```python
from build123d import *

# Parameters (mm, degrees)
SKETCH1_W               = 200
SKETCH1_H               = 100
BOSS_EXTRUDE1_DEPTH     = 2.6
FILLET1_R               = 10
SKETCH6_R               = 1.5
CUT_EXTRUDE6_DEPTH      = 2.6
MIRROR6_COPY_1_SKETCH_R = 1.5
MIRROR6_COPY_1_DEPTH    = 2.6
SKETCH15_R              = 10
CUT_EXTRUDE14_DEPTH     = 224.621913059
SKETCH20_R              = 1.27
CUT_EXTRUDE15_DEPTH     = 224.621913059
SKETCH23_R              = 1.524
CUT_EXTRUDE16_DEPTH     = 2.59999988
MIRROR8_COPY_1_SKETCH_R = 1.524
MIRROR8_COPY_1_DEPTH    = 2.59999988


with BuildPart() as part:
    # Sketch1 → Boss-Extrude1 (new body)
    with BuildSketch(Plane(origin=(0, 0, 0), x_dir=(1, 0, 0), z_dir=(0, 1, 0))):
        with Locations((100, -50)):
            Rectangle(SKETCH1_W, SKETCH1_H)
    extrude(amount=BOSS_EXTRUDE1_DEPTH)

    # Fillet1
    fillet1_edges = [part.edges().sort_by_distance(p)[0] for p in [
        (0, 1.3, 0),
        (200, 1.3, 0),
        (200, 1.3, 100),
        (0, 1.3, 100),
    ]]
    fillet(fillet1_edges, radius=FILLET1_R)

    # Sketch6 → Cut-Extrude6 (cut)
    with BuildSketch(Plane.XZ):
        with Locations(Location((190, 10, 0), (0, 0, 270))):
            Circle(SKETCH6_R)
    cut_extrude6 = extrude(amount=-CUT_EXTRUDE6_DEPTH, mode=Mode.SUBTRACT)

    # Mirror5: Cut-Extrude6 across plane
    add(cut_extrude6.mirror(Plane(origin=(100, 0, 0), x_dir=(0, 0, 1), z_dir=(1, 0, 0))), mode=Mode.SUBTRACT)

    # Mirror6: Cut-Extrude6 across plane
    add(cut_extrude6.mirror(Plane.XY.offset(50)), mode=Mode.SUBTRACT)

    # Mirror6 copy 1 sketch → Mirror6 copy 1 (cut)
    with BuildSketch(Plane(origin=(200, 0, 100), x_dir=(-1, 0, 0), z_dir=(0, -1, 0))):
        with Locations(Location((190, 10, 0), (0, 0, 270))):
            Circle(MIRROR6_COPY_1_SKETCH_R)
    extrude(amount=-MIRROR6_COPY_1_DEPTH, mode=Mode.SUBTRACT)

    # Sketch15 → Cut-Extrude14 (cut, through all)
    with BuildSketch(Plane.XZ):
        with Locations(Location((100, 50, 0), (0, 0, 270))):
            Circle(SKETCH15_R)
    extrude(amount=-CUT_EXTRUDE14_DEPTH, mode=Mode.SUBTRACT)

    # Sketch20 → Cut-Extrude15 (cut, through all)
    with BuildSketch(Plane(origin=(0, 2.6, 0), x_dir=(1, 0, 0), z_dir=(0, 1, 0))):
        with Locations(Location((158.41, -42.38, 0), (0, 0, 270))):
            Circle(SKETCH20_R)
        with Locations(Location((180, -42.38, 0), (0, 0, 270))):
            Circle(SKETCH20_R)
        with Locations(Location((158.41, -57.62, 0), (0, 0, 270))):
            Circle(SKETCH20_R)
        with Locations(Location((180, -57.62, 0), (0, 0, 270))):
            Circle(SKETCH20_R)
    extrude(amount=-CUT_EXTRUDE15_DEPTH, mode=Mode.SUBTRACT)

    # Sketch23 → Cut-Extrude16 (cut)
    with BuildSketch(Plane(origin=(0, 2.6, 0), x_dir=(1, 0, 0), z_dir=(0, 1, 0))):
        with Locations(Location((18.288, -9.906, 0), (0, 0, 270))):
            Circle(SKETCH23_R)
    cut_extrude16 = extrude(amount=-CUT_EXTRUDE16_DEPTH, mode=Mode.SUBTRACT)

    # Mirror7: Cut-Extrude16 across plane
    add(cut_extrude16.mirror(Plane(origin=(100, 0, 0), x_dir=(0, 0, 1), z_dir=(1, 0, 0))), mode=Mode.SUBTRACT)

    # Mirror8: Cut-Extrude16 across plane
    add(cut_extrude16.mirror(Plane.XY.offset(50)), mode=Mode.SUBTRACT)

    # Mirror8 copy 1 sketch → Mirror8 copy 1 (cut)
    with BuildSketch(Plane(origin=(200, 2.6, 100), x_dir=(-1, 0, 0), z_dir=(0, 1, 0))):
        with Locations(Location((18.288, -9.906, 0), (0, 0, 270))):
            Circle(MIRROR8_COPY_1_SKETCH_R)
    extrude(amount=-MIRROR8_COPY_1_DEPTH, mode=Mode.SUBTRACT)


solid = part.part
```
Check sheet for the modelled part. Datum: model origin and axes. Units: mm. Round coordinates to 2 decimals unless told otherwise and drop trailing zeros. Loops run counter-clockwise (first coordinate to the right, second up) from the corner with the lowest first, then second, coordinate; pieces in that order, holes last. Notation, with made-up numbers: (33.5, 44) - (50.5, 44) arc R38 ccw to (50.5, 83) - close; hole circle Ø9 at (-27.75, 55). An arc over 180 degrees is marked (long way). Write item = value, one per line. Start each with the question number.
Q1. Thickness scan on L1, parallel to X at y = 1.5, z = 10; L2, parallel to Z at x = 10, y = 1.5; L3, parallel to Z at x = 180, y = 1.75. Record the ranges inside material, lowest first.
Q2. Section check C-C (y = 1.6). Count the separate pieces of the cut face and the enclosed holes in it, plus the area to 3 significant figures.
Q3. Depth check by flat-ended pin: P1, Ø3.5, axis at x = 10, z = 90, coming from the -Y side; P2, Ø1.8, axis at x = 10, z = 10, coming from the -Y side. Enter the tip coordinate at first touch or a pass-through.
Q4. Section check B-B (z = 50). Record the boundary of the cut face in (x, y).
Q5. Release check for a two-part mould opening along Z. For faces 1 (the face through (2.85, 1.32, 96.99)), 2 (the face through (109.915, 1.282, 51.302)), 3 (the face through (99, 0, 38)) record: pulls with the +Z half, pulls with the -Z half, needs draft (parallel to the pull), parting line crosses it, or undercut.
Q6. Section check A-A (x = 100). Record the boundary of the cut face in (y, z), plus the area to 3 significant figures.
Derived:
q1.L1 = 0 to 8.5, 11.5 to 16.77, 19.81 to 180.19, 183.23 to 188.5, 191.5 to 200
q1.L2 = 0 to 8.5, 11.5 to 88.5, 91.5 to 100
q1.L3 = 0 to 41.11, 43.65 to 56.35, 58.89 to 100
q2.separate_pieces = 1
q2.enclosed_holes = 13
q2.area = 19,500 mm^2
q3.P1 = 0
q3.P2 = through
q4.outline = (0, 0) - (90, 0) - (90, 2.6) - (0, 2.6) - close; (110, 0) - (200, 0) - (200, 2.6) - (110, 2.6) - close
q5.face_1 = pulls with the +Z half
q5.face_2 = undercut
q5.face_3 = needs draft
q6.outline = (0, 0) - (2.6, 0) - (2.6, 40) - (0, 40) - close; (0, 60) - (2.6, 60) - (2.6, 100) - (0, 100) - close
q6.area = 208 mm^2
